Here's the drawing with two shaded views (mm, measured from the low corner). I have some questions. A direction names the side the tool comes from. Round coordinates to 2 decimals unless told otherwise and drop trailing zeros. Loops run counter-clockwise (first coordinate to the right, second up) from the corner with the lowest first, then second, coordinate; pieces in that order, holes last. Notation, with made-up numbers: M 3,66 L 39,66 A26 ccw 39,105 Z; hole C -7.75,45.25 d3. An arc over 180 degrees is marked long. Write each question's results on one line, items separated by ' | '. Start each with the question number.
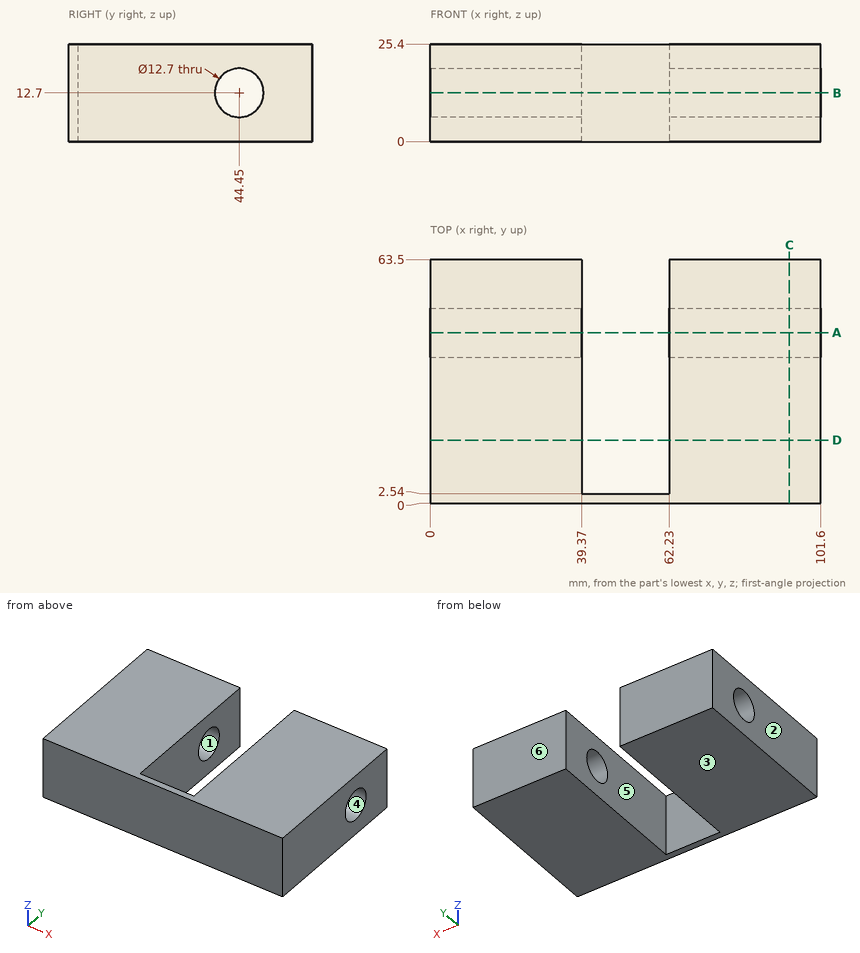
Item 1: I need wall thicknesses on L1, parallel to Y at x = 87, z = 12.7; L2, parallel to X at y = 56.5, z = 19; L3, parallel to Z at x = 85, y = 44. Which ranges of each line are inside material? Lowest first, please.
Item 2: If we section it at C-C on x = 93.5: Please give me the cut outline in (y, z).
Item 3: If we section it at B-B on z = 12.7: Please give me the cut outline in (x, y).
Item 4: If we section it at D-D on y = 16.5: Please give me the cut outline in (x, z).
Item 5: If we mould it in two halves opening along Z, with no side actions, what happens to the marked faces 1, 2, 3 and 4? For each: released by +Z, released by -Z, zero draft, split by the parting line, or undercut.
Item 6: Which directions (+Z, -Z, +X, -X, +Y, -Y) give clear straight access to the entire face, cutting with the end or side of a thin tool? Please do the marked faces 5 and 6.
Item 7: If we section it at A-A on y = 44.45: Please give me the cut outline in (x, z), and give its area (4 significant figures).
Numbers:
1) L1: 0 to 38.1, 50.8 to 63.5 | L2: 0 to 39.37, 62.23 to 101.6 | L3: 0 to 6.37, 19.03 to 25.4
2) outline: M 0,0 L 63.5,0 L 63.5,25.4 L 0,25.4 Z; hole C 44.45,12.7 d12.7
3) outline: M 0,0 L 101.6,0 L 101.6,38.1 L 62.23,38.1 L 62.23,2.54 L 39.37,2.54 L 39.37,38.1 L 0,38.1 Z; M 0,50.8 L 39.37,50.8 L 39.37,63.5 L 0,63.5 Z; M 62.23,50.8 L 101.6,50.8 L 101.6,63.5 L 62.23,63.5 Z
4) outline: M 0,0 L 39.37,0 L 39.37,25.4 L 0,25.4 Z; M 62.23,0 L 101.6,0 L 101.6,25.4 L 62.23,25.4 Z
5) face 1: undercut | face 2: zero draft | face 3: released by -Z | face 4: undercut
6) face 5: +Z, -Z, +Y | face 6: +Z, -Z, +X, -X, +Y
7) outline: M 0,0 L 39.37,0 L 39.37,6.35 L 0,6.35 Z; M 0,19.05 L 39.37,19.05 L 39.37,25.4 L 0,25.4 Z; M 62.23,0 L 101.6,0 L 101.6,6.35 L 62.23,6.35 Z; M 62.23,19.05 L 101.6,19.05 L 101.6,25.4 L 62.23,25.4 Z | area: 1,000 mm²
